Geometry check sheet. Reference: drawing and pictorial views, mm from the part's lowest x, y, z. A direction names the side the tool comes from. Round coordinates to 2 decimals unless told otherwise and drop trailing zeros. Order: outer loops, then holes, each group sorted by start corner. A loop starts at its lowest first (then second) coordinate and runs counter-clockwise, first axis right, second up.
(1) Set-up check for the marked faces 1, 2 and 3: record each of +Z, -Z, +X, -X, +Y, -Y from which the full face is reachable in a straight line by a thin tool's end or side.
(2) Gauge pin test, flat ends, axial feed: P1, Ø2, axis at x = 21, y = 7.5, coming from the -Z side; P2, Ø2, axis at x = 87.5, z = 2.5, coming from the -Y side; P3, Ø1.5, axis at y = 8.5, z = 1.5, coming from the -X side. Record the tip position at first contact, or that the pin passes through.
(3) Cross-section at B-B on z = 4.5. Enter the section's corners in (x, y) (1 decimal).
(4) Cross-section at C-C on x = 142.5. Enter the section's corners in (y, z).
(5) Cross-section at A-A on y = 7.75. Enter the section's corners in (x, z).
(6) Thickness scan on L1, parallel to X at y = 3, z = 7.75; L2, parallel to X at y = 11.5, z = 8.5; L3, parallel to Y at x = 90, z = 6.5. Record the ranges inside material, lowest first.
(7) Cross-section at D-D on x = 93. Enter the section's corners in (y, z).
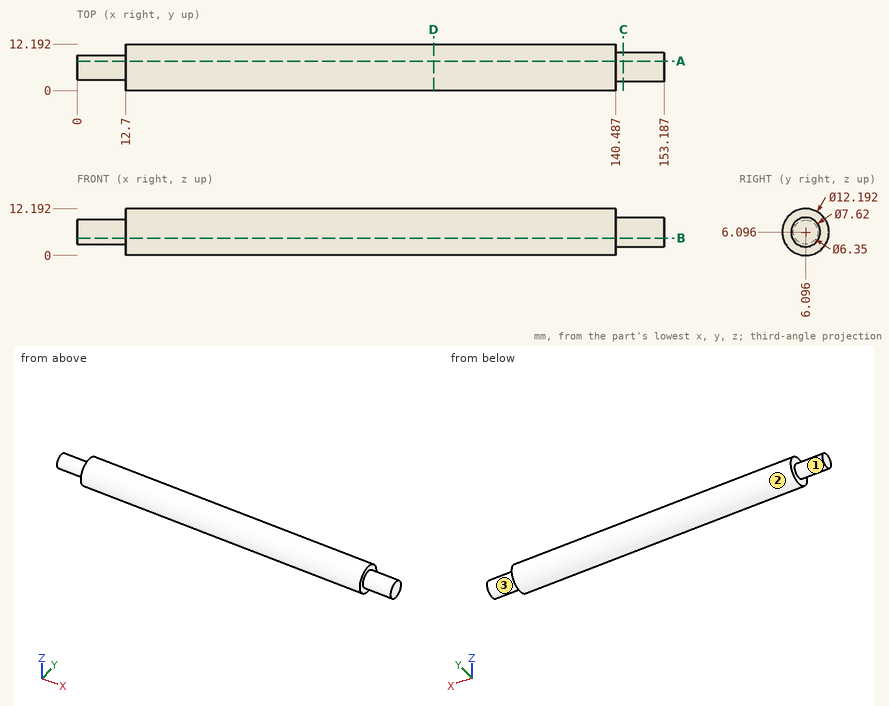
Found:
1. face 1: -X
1. face 2: +X, -X
1. face 3: +X
2. P1: stops at z = 0.01
2. P2: stops at y = 0.58
2. P3: stops at x = 12.7
3. outline: (0, 3.4) - (12.7, 3.4) - (12.7, 0.2) - (140.5, 0.2) - (140.5, 2.6) - (153.2, 2.6) - (153.2, 9.6) - (140.5, 9.6) - (140.5, 12) - (12.7, 12) - (12.7, 8.8) - (0, 8.8) - close
4. outline: circle Ø7.62 at (6.1, 6.1)
5. outline: (0, 3.39) - (12.7, 3.39) - (12.7, 0.23) - (140.49, 0.23) - (140.49, 2.66) - (153.19, 2.66) - (153.19, 9.53) - (140.49, 9.53) - (140.49, 11.96) - (12.7, 11.96) - (12.7, 8.81) - (0, 8.81) - close
6. L1: x = 12.7 to 153.19
6. L2: x = 12.7 to 140.49
6. L3: y = 0.01 to 12.18
7. outline: circle Ø12.19 at (6.1, 6.1)
